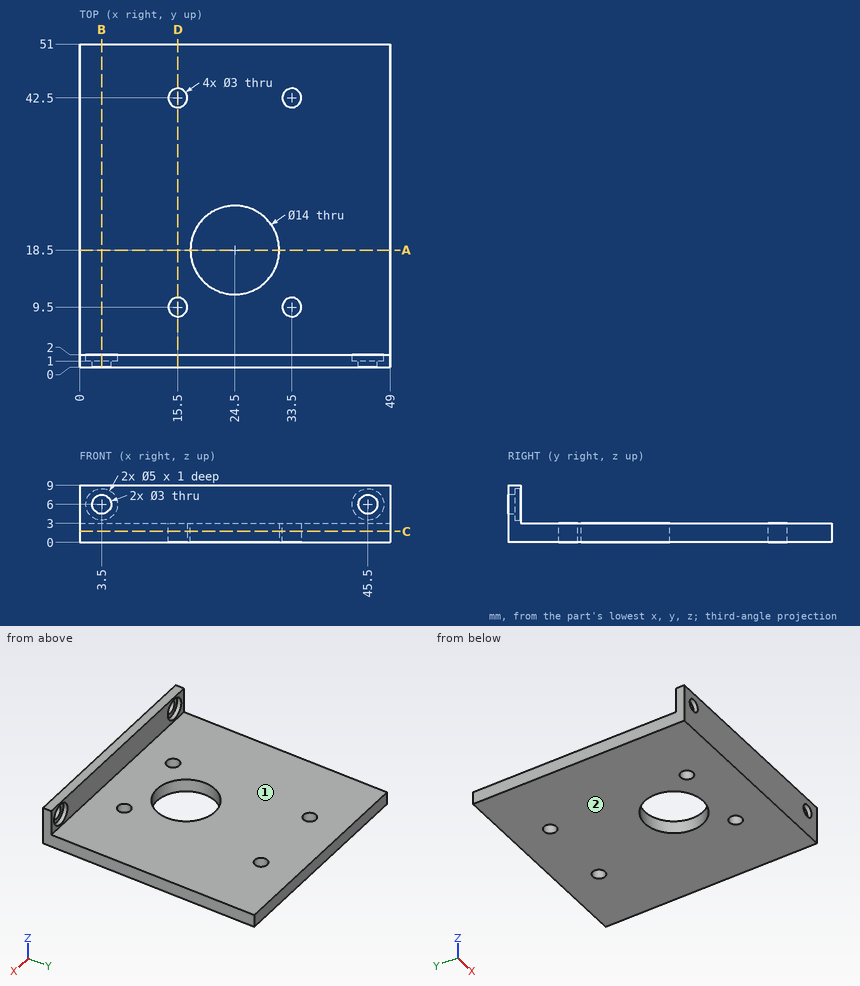
The drawing under review shows one solid part. Ordinate dimensions are in mm from its lowest x, y, z. A direction names the side the tool comes from. Give positions to 0.01 mm unless a question says otherwise; leave off trailing zeros. Write each loop counter-clockwise with the first axis right and the second up, starting at its lowest first coordinate (ties: lowest second). Pieces come first, ordered by that corner, then holes.
1. Tool access review of the marked faces 1 and 2: name each direction out of +Z, -Z, +X, -X, +Y, -Y from which nothing blocks a thin tool from reaching the whole face with its end or side.
2. Add section D-D, the plane x = 15.5. Write out the cut boundary in (y, z).
3. Wall thickness on L1, parallel to X at y = 0.5, z = 6; L2, parallel to Y at x = 15.5, z = 2.4; L3, parallel to Y at x = 24.5, z = 2.25: over which ranges is each line inside the solid? List them lowest first.
4. Add section A-A, the plane y = 18.5. Write out the cut boundary in (x, z).
5. Add section B-B, the plane x = 3.5. Write out the cut boundary in (y, z).
6. For P1, Ø16, axis at x = 24.5, y = 18.5, coming from the +Z side; P2, Ø1.5, axis at x = 46, z = 5, coming from the +Y side; P3, Ø1.8, axis at x = 17.5, z = 6, coming from the +Y side; P4, Ø1.8, axis at x = 33.5, y = 42.5, coming from the +Z side, all flat-tipped, find the tip position at first contact; note any pin that passes through.
7. Add section C-C, the plane z = 1.75. Write out the cut boundary in (x, y), plus the area to 3 significant figures.
Worked answers:
1. face 1: +Z, +X, -X, +Y
1. face 2: -Z, +X, -X, +Y, -Y
2. outline: (0, 0) - (8, 0) - (8, 3) - (2, 3) - (2, 9) - (0, 9) - close; (11, 0) - (41, 0) - (41, 3) - (11, 3) - close; (44, 0) - (51, 0) - (51, 3) - (44, 3) - close
3. L1: x = 0 to 2, 5 to 44, 47 to 49
3. L2: y = 0 to 8, 11 to 41, 44 to 51
3. L3: y = 0 to 11.5, 25.5 to 51
4. outline: (0, 0) - (17.5, 0) - (17.5, 3) - (0, 3) - close; (31.5, 0) - (49, 0) - (49, 3) - (31.5, 3) - close
5. outline: (0, 0) - (51, 0) - (51, 3) - (2, 3) - (2, 3.5) - (1, 3.5) - (1, 4.5) - (0, 4.5) - close; (0, 7.5) - (1, 7.5) - (1, 8.5) - (2, 8.5) - (2, 9) - (0, 9) - close
6. P1: stops at z = 3
6. P2: stops at y = 1
6. P3: stops at y = 2
6. P4: passes through
7. outline: (0, 0) - (49, 0) - (49, 51) - (0, 51) - close; hole circle Ø3 at (15.5, 9.5); hole circle Ø3 at (15.5, 42.5); hole circle Ø14 at (24.5, 18.5); hole circle Ø3 at (33.5, 9.5); hole circle Ø3 at (33.5, 42.5)
7. area: 2,320 mm2
